Study the drawing (mm; zero at the part's minimum x, y, z) and answer. A direction names the side the tool comes from. Give positions to 0.01 mm unless a question says otherwise; leave off trailing zeros. Order: outer loops, then holes, each group sorted by start corner. A loop starts at its lowest first (then second) coordinate and runs counter-clockwise, first axis right, second up. Notation, with made-up numbers: (65.25, 55.25) - (83.25, 55.25) arc R15 cw to (83.25, 62.25) - close; hole circle Ø7 at (-37.5, -7.5). An arc over 180 degrees is marked (long way). Write each question's results on one line, items separated by ' | '. Start each with the question number.
Q1. For a pull along Z with two mould halves and no side action, classify the marked faces 1, 2 and 3 as +Z half, -Z half, draft (parallel to the pull), parting line (faces both ways), or undercut.
Q2. Find the intervals of material crossed by line 1 along Z through (x, y) = (22, 18) (3 decimals); line 2 along Y through (x, z) = (12.7, 8.5); line 3 along Y through (x, z) = (13.25, 9.5), in increasing order. Write a range as from..to.
Q3. Flat-ended cylindrical pins translate along their axes: P1, Ø6, axis at y = 8.5, z = 2, coming from the -X side; P2, Ø5, axis at y = 9.5, z = 6.5, coming from the -X side; P3, Ø3, axis at y = 22, z = 2.5, coming from the +X side. Find the tip coordinate at first contact, or state that the pin passes through.
Q4. Find section A-A on y = 12.7. Give the vertices of the cut face in (x, z) (3 decimals).
Q5. Find section C-C on x = 2. Give the vertices of the cut face in (y, z) (3 decimals), and give its area (3 significant figures).
Q6. Find section D-D on z = 8.25. Give the vertices of the cut face in (x, y).
Q7. A tool of negligible diameter and unlimited length cuts with its end or side. For the marked faces 4 and 5, from which of +Z, -Z, +X, -X, +Y, -Y can it reach the whole face along a straight path? Write none if from no direction.
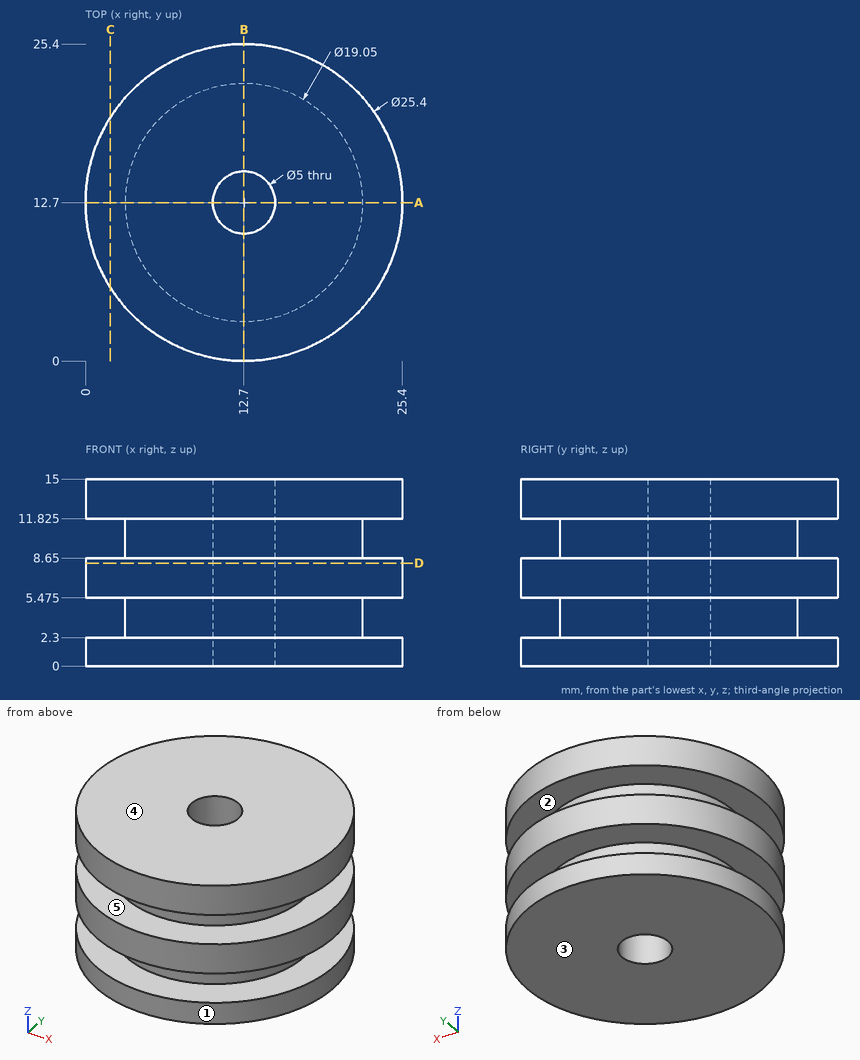
Working result:
1) face 1: draft | face 2: undercut | face 3: -Z half
2) line 1: 0..2.3, 5.475..8.65, 11.825..15 | line 2: 0..10.2, 15.2..25.4 | line 3: 3.19..10.26, 15.14..22.21
3) P1: x = 0.06 | P2: x = 0.02 | P3: x = 22.71
4) outline: (0, 0) - (10.2, 0) - (10.2, 15) - (0, 15) - (0, 11.825) - (3.175, 11.825) - (3.175, 8.65) - (0, 8.65) - (0, 5.475) - (3.175, 5.475) - (3.175, 2.3) - (0, 2.3) - close; (15.2, 0) - (25.4, 0) - (25.4, 2.3) - (22.225, 2.3) - (22.225, 5.475) - (25.4, 5.475) - (25.4, 8.65) - (22.225, 8.65) - (22.225, 11.825) - (25.4, 11.825) - (25.4, 15) - (15.2, 15) - close
5) outline: (5.859, 0) - (19.541, 0) - (19.541, 2.3) - (5.859, 2.3) - close; (5.859, 5.475) - (19.541, 5.475) - (19.541, 8.65) - (5.859, 8.65) - close; (5.859, 11.825) - (19.541, 11.825) - (19.541, 15) - (5.859, 15) - close | area: 118 mm²
6) outline: circle Ø25.4 at (12.7, 12.7); hole circle Ø5 at (12.7, 12.7)
7) face 4: +Z, +X, -X, +Y, -Y | face 5: none
